Part model, mm, in its own coordinate system. A direction names the side the tool comes from. Round coordinates to 2 decimals unless told otherwise and drop trailing zeros. Loops run counter-clockwise (first coordinate to the right, second up) from the corner with the lowest first, then second, coordinate; pieces in that order, holes last. Notation, with made-up numbers: M 23.25,76.5 L 82.25,76.5 A15 cw 82.25,91.5 Z; hole C 2.25,-36.75 d7. An arc over 180 degrees is marked long. Put each result on its own line as item: value. Start each with the question number.
1) Probe line 1 along Y through (x, z) = (21.5, -0.3); line 2 along Y through (x, z) = (18, -0.25). List the from-to ranges inside material, lowest first.
2) Drop a flat-ended pin along its axis: pin 1 Ø1 at (x, z) = (-5, -1) entering from +Y. Give the stop position or say it passes through.
3) Slice it at B-B on x = -10.5. Give the cut face in (y, z), then the cut area to 3 significant figures.
4) Slice it at A-A on z = -0.45. State how many separate pieces and enclosed holes the cut face has, then the cut area to 3 significant figures.
5) Which spindle directions (+Z, -Z, +X, -X, +Y, -Y) get a long thin tool onto all of the face, cutting with end or side? Do faces 1 (the flat face through (0, 2, 0)), 2 (the flat face through (6, 21.2, -1)). Say none if no direction does.
Autodesk Inventor part; units mm, degrees
ref_plane "Plano de trabajo1" through (0, 0, -1.6) normal (0, 0, 1) x (1, 0, 0)
ref_plane "YZ Plane" through (0, 0, 0) normal (1, 0, 0) x (0, 1, 0)
ref_plane "XZ Plane" through (0, 0, 0) normal (0, 1, 0) x (-1, 0, 0)
sketch "Boceto1" plane through (0, 0, 0) normal (0, 0, 1) x (1, 0, 0)
  line L0 (-26, 26) -> (26, 26)
  line L1 (26, 26) -> (26, -26)
  line L2 (26, -26) -> (-26, -26)
  line L3 (-26, -26) -> (-26, 26)
  line L4 (-26, 26) -> (26, -26) construction
  line L5 (26, 26) -> (-26, -26) construction
  point P0 (0, 0)
  dimension "d0" = 52
  dimension "d1" = 52
extrude "Extrusión1" add sketch "Boceto1" against normal blind 1.742
fillet "Empalme1" radius 0.5 4 edges at (26, 26, -0.871) (-26, 26, -0.871) (-26, -26, -0.871) (26, -26, -0.871)
ref_plane "Plano de trabajo1" through (0, 0, -1.6) normal (0, 0, 1) x (1, 0, 0)
sketch "Boceto6" plane through (0, 0, 0) normal (0, 0, 1) x (1, 0, 0)
  line L0 (-25.5, 26) -> (25.5, 26) construction
  line L1 (-25.5, 26) -> (25.5, 26) construction
  line L2 (-15.5, 26) -> (26, 26)
  line L3 (26, 26) -> (26, 21.2)
  line L4 (26, 21.2) -> (-15.5, 21.2)
  line L5 (-15.5, 21.2) -> (-15.5, 26)
  line L6 (26, 25.5) -> (26, -25.5)
  point P0 (0, 0)
  dimension "d14" = 4.8
  dimension "d15" = 41.5
extrude "Extrusión4" cut sketch "Boceto6" against normal through all
sketch "Boceto7" plane through (0, 0, -1.742) normal (0, 0, -1) x (-1, 0, 0)
  line L0 (25.5, 26) -> (15.5, 26)
  arc A0 (26, 25.5) -> (25.5, 26) centre (25.5, 25.5) ccw
  line L1 (26, 25.5) -> (26, 28.5)
  line L2 (26, 28.5) -> (15.5, 28.5)
  line L3 (15.5, 28.5) -> (15.5, 26)
  point P0 (0, 0)
  dimension "d18" = 2.5
extrude "Extrusión5" add sketch "Boceto7" against normal up to surface (1.742 mm away)
sketch "Boceto9" plane through (0, 0, -1.742) normal (0, 0, -1) x (-1, 0, 0)
  circle A0 centre (-21.765, -9.26) radius 0.37
  circle A1 centre (-23.035, -9.26) radius 0.37
  circle A2 centre (-23.035, -10.53) radius 0.37
  circle A3 centre (-21.765, -10.53) radius 0.37
  circle A4 centre (-23.035, -11.8) radius 0.37
  circle A5 centre (-21.765, -11.8) radius 0.37
  circle A6 centre (-23.035, -13.07) radius 0.37
  circle A7 centre (-21.765, -13.07) radius 0.37
  circle A8 centre (-23.035, -14.34) radius 0.37
  circle A9 centre (-21.765, -14.34) radius 0.37
  point P0 (0, 0)
extrude "Extrusión6" cut sketch "Boceto9" against normal up to surface (1.742 mm away)
fillet "Empalme2" radius 0.5 4 edges at (26, 21.2, -0.871) (-15.5, 21.2, -0.871) (-15.5, 28.5, -0.871) (-26, 28.5, -0.871)
properties part number "hw_DAA - PCB Power" material "PCB"
Recorded:
1. line 1: y = -26 to -14.6, -14.08 to -13.33, -12.81 to -12.06, -11.54 to -10.79, -10.27 to -9.52, -9 to 21.2
1. line 2: y = -26 to 21.2
2. pin 1: stops at y = 21.2
3. outline: M -26,-1.74 L 21.2,-1.74 L 21.2,0 L -26,0 Z
3. area: 82.2 mm2
4. separate pieces: 1
4. enclosed holes: 10
4. area: 2,530 mm2
5. face 1: +Z, +X, -X, +Y, -Y
5. face 2: +Z, -Z, +X, +Y
